from build123d import *

# Parameters (mm, degrees)
F1_DEPTH = 12.7
F2_W     = 2.54
F2_H     = 3.937
F3_DEPTH = 25.4
F4_R     = 1.524


with BuildPart() as f1:
    # F0 (on Front) → F1 (new body)
    with BuildSketch(Plane.XZ):
        Polygon((-2.863529, 1.524), (-3.743411, 0), (3.622589, 0), (2.742708, 1.524), (5.488804, 1.524), (5.488804, 5.461), (-5.609625, 5.461), (-5.609625, 1.524), align=None)
    extrude(amount=F1_DEPTH)

    # F2 (on face) → F3 (intersect)
    with BuildSketch(Plane.YZ.offset(5.488804)):
        with Locations((-6.35, 3.4925)):
            Rectangle(F2_W, F2_H)
        Polygon((-7.62, 1.524), (-12.7, 1.524), (-12.7, 0), (0, 0), (0, 1.524), (-5.08, 1.524), align=None)
    extrude(amount=-F3_DEPTH, mode=Mode.INTERSECT)

    # F4
    f4_edges = [f1.edges().sort_by_distance(p)[0] for p in [
        (-5.609625, -6.35, 5.461),
    ]]
    fillet(f4_edges, radius=F4_R)


solid = f1.part
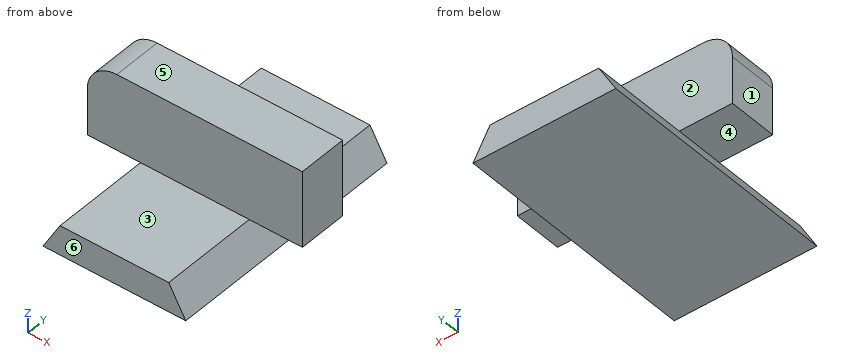
Input: part model. Units: mm. Frame: model coordinates. Face numbers are marked on the shaded views. A direction names the side the tool comes from. Coordinates: 2 decimals unless noted, no trailing zeros. Loops run counter-clockwise (first coordinate to the right, second up) from the corner with the lowest first, then second, coordinate; pieces in that order, holes last. Notation, with made-up numbers: (-9, 34) -> (-4, 34) arc R28 ccw to (-4, 61) -> close; hole circle Ø3 at (38, 37). An arc over 180 degrees is marked (long way). One line per item, written item: value.
(1) Cut plane A-A (x = -1.5). Output: boundary loops of the cut face in (y, z).
Answer below:
outline: (-12.7, 0) -> (0, 0) -> (0, 1.52) -> (-5.08, 1.52) -> (-5.08, 5.46) -> (-7.62, 5.46) -> (-7.62, 1.52) -> (-12.7, 1.52) -> close
(2) Cut plane B-B (y = -3.25). Output: boundary loops of the cut face in (x, z).
Answer below:
outline: (-3.74, 0) -> (3.62, 0) -> (2.74, 1.52) -> (-2.86, 1.52) -> close
(3) Draft query along Z for the marked faces 4, 5 and 6. Return one class per face: pulls with the +Z half, pulls with the -Z half, needs draft (parallel to the pull), parting line crosses it, or undercut.
Answer below:
face 4: undercut
face 5: pulls with the +Z half
face 6: needs draft
(4) Set-up query: the marked faces 1, 2 and 3. Return all of +Z, -Z, +X, -X, +Y, -Y with unobstructed straight access to the full face (end or side cutting, diameter ignored); none if empty.
Answer below:
face 1: +Z, -Z, -X, +Y, -Y
face 2: +Z, +X, -X, +Y
face 3: +Z, +X, -X, -Y
(5) Pin query (flat end, axial travel): pin 1 Ø3 at (x, y) = (-3, -9.5) entering from +Z; pin 2 Ø1.2 at (x, z) = (1, 4) entering from +Y; pin 3 Ø1.2 at (x, z) = (-0.5, 4) entering from -Y. Return the tip coordinate at first contact, or that it passes through.
Answer below:
pin 1: stops at z = 1.52
pin 2: stops at y = -5.08
pin 3: stops at y = -7.62
(6) Cut plane C-C (z = 2.05). Output: boundary loops of the cut face in (x, y), then the cut area to 3 significant figures.
Answer below:
outline: (-5.61, -7.62) -> (5.49, -7.62) -> (5.49, -5.08) -> (-5.61, -5.08) -> close
area: 28.2 mm2
(7) Ray query, line 1 along Y through (x, z) = (0.75, 2.25); line 2 along Z through (x, y) = (2.5, -3); line 3 along X through (y, z) = (-6.75, 4.2). Return the intervals inside material, ascending.
Answer below:
line 1: y = -7.62 to -5.08
line 2: z = 0 to 1.52
line 3: x = -5.59 to 5.49
